Read the model definition and answer for the solid it produces. Units are mm, in the model's axes. Face numbers are marked on the shaded views. A direction names the side the tool comes from. Round coordinates to 2 decimals unless told otherwise and drop trailing zeros. Order: outer loops, then holes, each group sorted by start corner. A loop starts at its lowest first (then second) coordinate and runs counter-clockwise, first axis right, second up. Notation, with made-up numbers: (62, 10.25) -> (88, 10.25) arc R21 cw to (88, 45.25) -> close; hole circle Ø6 at (-6, -5). An arc over 180 degrees is marked (long way). Answer as a JSON object with one key per item and string values. Group by question number.
Item 1: Section C-C, the plane x = 22.5 is taken. Write down the section's boundary in (y, z).
Item 2: Section D-D, the plane z = -1 is taken. Count the separate pieces of the cut face and the enclosed holes in it, plus the area to 3 significant figures.
Item 3: For the marked faces 1, 2 and 3, determine the directions among +Z, -Z, +X, -X, +Y, -Y from which every point of the face is accessible in a straight line to the end or side of a thin tool.
Item 4: Section B-B, the plane y = 65.8 is taken. Write down the section's boundary in (x, z).
Item 5: Consider probe 1 along Y at (x, z) = (0, 2.5); probe 2 along Y at (x, z) = (-38, -2.75); probe 3 along Y at (x, z) = (22.5, -2.75). Determine where each line is inside the solid, lowest interval first. Write a range as from..to.
Item 6: Section A-A, the plane x = -42.5 is taken. Write down the section's boundary in (y, z), plus the area to 3 significant figures.
Item 7: Given P1, Ø6, axis at y = 58.5, z = 2, coming from the +X side; P2, Ø1.5, axis at x = -33.5, z = -3, coming from the +Y side; P3, Ø5, axis at y = 16.5, z = 3, coming from the -X side, each flat-ended and moving along its own axis, determine where each tip first touches the part or whether it passes through.
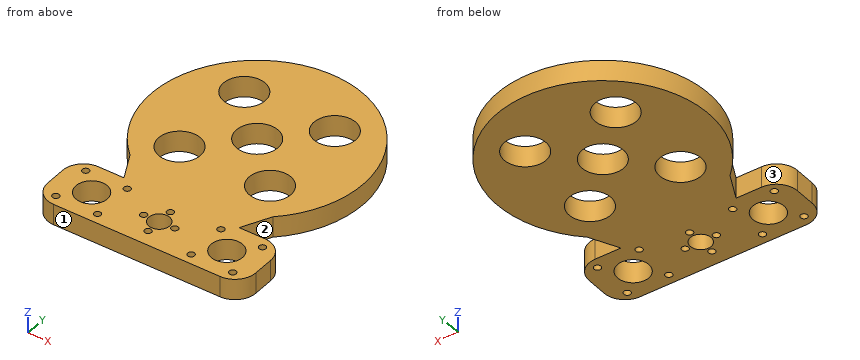
Autodesk Inventor part; units mm, degrees
ref_plane "YZ Plane" through (0, 0, 0) normal (1, 0, 0) x (0, 1, 0)
ref_plane "XZ Plane" through (0, 0, 0) normal (0, 1, 0) x (-1, 0, 0)
ref_plane "XY Plane" through (0, 0, 0) normal (0, 0, 1) x (1, 0, 0)
sketch "Sketch1" plane through (0, 0, 0) normal (0, 0, 1) x (1, 0, 0)
  line L0 (-50, -15) -> (50, -15)
  line L1 (50, -15) -> (50, 15)
  line L2 (50, 15) -> (-50, 15)
  line L3 (-50, 15) -> (-50, -15)
  line L4 (-50, -15) -> (50, 15) construction
  line L5 (50, -15) -> (-50, 15) construction
  line L6 (-42.5, 10) -> (-22.5, 10) construction
  line L7 (-22.5, 10) -> (-22.5, -10) construction
  line L8 (-22.5, -10) -> (-42.5, -10) construction
  line L9 (-42.5, -10) -> (-42.5, 10) construction
  line L10 (-42.5, 10) -> (-22.5, -10) construction
  line L11 (-22.5, 10) -> (-42.5, -10) construction
  line L12 (0, 0) -> (0, 8.2744) construction
  circle A0 centre (0, 0) radius 5
  circle A1 centre (-42.5, 10) radius 1.65
  circle A2 centre (-22.5, 10) radius 1.65
  circle A3 centre (-22.5, -10) radius 1.65
  circle A4 centre (-42.5, -10) radius 1.65
  circle A5 centre (-32.5, 0) radius 7.5
  line L13 (0, 0) -> (0, 9.2231)
  line L14 (42.5, 10) -> (22.5, 10) construction
  line L15 (22.5, 10) -> (22.5, -10) construction
  line L16 (22.5, -10) -> (42.5, -10) construction
  line L17 (42.5, -10) -> (42.5, 10) construction
  line L18 (42.5, 10) -> (22.5, -10) construction
  line L19 (22.5, 10) -> (42.5, -10) construction
  circle A6 centre (42.5, 10) radius 1.65
  circle A7 centre (22.5, 10) radius 1.65
  circle A8 centre (22.5, -10) radius 1.65
  circle A9 centre (42.5, -10) radius 1.65
  circle A10 centre (32.5, 0) radius 7.5
  circle A11 centre (0, 7.5) radius 1.65
  circle A12 centre (-7.5, 0) radius 1.65
  circle A13 centre (0, -7.5) radius 1.65
  circle A14 centre (7.5, 0) radius 1.65
  point P0 (-9.2231, 0)
  point P1 (0, -9.2231)
  point P2 (9.2231, 0)
  dimension "d0" = 10
  dimension "d1" = 3.3
  dimension "d2" = 32.5
  dimension "d3" = 20
  dimension "d4" = 20
  dimension "d5" = 15
  dimension "d6" = 3.3
  dimension "d7" = 7.5
  dimension "d10" = 360
  dimension "d12" = 30
  dimension "d13" = 100
extrude "Extrusion1" add sketch "Sketch1" along normal mid plane 10
sketch "Sketch2" plane through (0, 0, 0) normal (0, 0, 1) x (1, 0, 0)
  circle A0 centre (0, 65.8) radius 50.8
  line L0 (50, -15) -> (50, 15)
  line L1 (50, 15) -> (-50, 15)
  line L2 (-50, 15) -> (-50, -15)
  line L3 (-50, -15) -> (50, -15)
  circle A1 centre (0, 0) radius 5
  circle A2 centre (7.5, 0) radius 1.65
  circle A3 centre (-7.5, 0) radius 1.65
  circle A4 centre (22.5, 10) radius 1.65
  circle A5 centre (42.5, 10) radius 1.65
  circle A6 centre (-42.5, 10) radius 1.65
  circle A7 centre (-22.5, 10) radius 1.65
  circle A8 centre (-22.5, -10) radius 1.65
  circle A9 centre (-42.5, -10) radius 1.65
  circle A10 centre (-32.5, 0) radius 7.5
  circle A11 centre (22.5, -10) radius 1.65
  circle A12 centre (32.5, 0) radius 7.5
  circle A13 centre (42.5, -10) radius 1.65
  circle A14 centre (0, 7.5) radius 1.65
  circle A15 centre (0, -7.5) radius 1.65
  line L4 (50, 15) -> (-50, 15)
  line L5 (-34.3016, 28.3294) -> (-27.6889, 15)
  line L6 (0, 15) -> (0, 36.3785)
  line L7 (34.3016, 28.3294) -> (27.6889, 15)
  circle A16 centre (-21.7564, 87.5564) radius 10
  circle A17 centre (-21.7564, 44.0436) radius 10
  circle A18 centre (21.7564, 44.0436) radius 10
  circle A19 centre (21.7564, 87.5564) radius 10
  line L8 (-21.7564, 44.0436) -> (21.7564, 44.0436) construction
  line L9 (21.7564, 44.0436) -> (21.7564, 87.5564) construction
  line L10 (21.7564, 87.5564) -> (-21.7564, 87.5564) construction
  line L11 (-21.7564, 87.5564) -> (-21.7564, 44.0436) construction
  line L12 (-21.7564, 44.0436) -> (21.7564, 87.5564) construction
  line L13 (21.7564, 44.0436) -> (-21.7564, 87.5564) construction
  circle A20 centre (0, 65.8) radius 10
  point P0 (-27.6889, 15)
  point P1 (27.6889, 15)
  dimension "d16" = 101.6
  dimension "d17" = 20
extrude "Extrusion2" add sketch "Sketch2" along normal mid plane 10 contours A0 | A0 L1 L5 | L7 L1 A0
fillet "Fillet1" radius 10 4 edges at (-50, -15, 0) (-50, 15, 0) (50, 15, 0) (50, -15, 0)
properties part number "APLASTADOR" material "Steel, Mild, Welded"
Values found:
{
 "1": {"outline": "(-15, -5) -> (-11.65, -5) -> (-11.65, 5) -> (-15, 5) -> close; (-8.35, -5) -> (8.35, -5) -> (8.35, 5) -> (-8.35, 5) -> close; (11.65, -5) -> (34.07, -5) -> (34.07, 5) -> (11.65, 5) -> close; (54.02, -5) -> (77.58, -5) -> (77.58, 5) -> (54.02, 5) -> close; (97.53, -5) -> (111.35, -5) -> (111.35, 5) -> (97.53, 5) -> close"},
 "2": {"separate pieces": "1", "enclosed holes": "20", "area": "9,110 mm2"},
 "3": {"face 1": "+Z, -Z, +X, -X, -Y", "face 2": "+Z, -Z, +X", "face 3": "+Z, -Z, -X"},
 "4": {"outline": "(-50.8, -5) -> (-10, -5) -> (-10, 5) -> (-50.8, 5) -> close; (10, -5) -> (50.8, -5) -> (50.8, 5) -> (10, 5) -> close"},
 "5": {"probe 1": "-15..-9.15, -5.85..-5, 5..5.85, 9.15..55.8, 75.8..116.6", "probe 2": "-15..-5.1, 5.1..15, 32.09..99.51", "probe 3": "-15..-11.65, -8.35..8.35, 11.65..34.07, 54.02..77.58, 97.53..111.35"},
 "6": {"outline": "(-14.68, -5) -> (-11.65, -5) -> (-11.65, 5) -> (-14.68, 5) -> close; (-8.35, -5) -> (8.35, -5) -> (8.35, 5) -> (-8.35, 5) -> close; (11.65, -5) -> (14.68, -5) -> (14.68, 5) -> (11.65, 5) -> close; (37.97, -5) -> (93.63, -5) -> (93.63, 5) -> (37.97, 5) -> close", "area": "784 mm2"},
 "7": {"P1": "x = 50.62", "P2": "y = 104.63", "P3": "x = -44.36"}
}
